Geometry check sheet. Reference: the model listing, model coordinates, mm. Face numbers are marked on the shaded views. A direction names the side the tool comes from. Coordinates: 2 decimals unless noted, no trailing zeros. Order: outer loops, then holes, each group sorted by start corner. A loop starts at its lowest first (then second) coordinate and runs counter-clockwise, first axis right, second up. Notation, with made-up numbers: M 46.25,-38.75 L 88.25,-38.75 A23 cw 88.25,-25.75 Z; hole C 30.5,-19.75 d10. An arc over 180 degrees is marked long. One line per item, written item: value. Start each with the question number.
1) Access from +Z, -Z, +X, -X, +Y, -Y to the whole of each face (thin tool, end or side, straight path). Record for the marked faces 1 and 2.
2) Go/stop test with flat-tipped pins: P1, Ø1, axis at x = -11, z = 11, coming from the -Y side; P2, Ø1, axis at y = 55.5, z = 3, coming from the +X side; P3, Ø7, axis at x = -10.5, z = 8.5, coming from the -Y side; P4, Ø8, axis at x = 5, y = 83, coming from the -Z side. Record where each tip stops, or that it passes through.
3) Draft check along Y on the marked faces 3, 4 and 5. Enter one of: pulls with the +Y half, pulls with the -Y half, needs draft (parallel to the pull), parting line crosses it, or undercut.
4) Sectioned sample at D-D, the plane y = 89. Enter the section's corners in (x, z), then the cut area to 3 significant figures.
5) Sectioned sample at B-B, the plane y = 49. Enter the section's corners in (x, z), then the cut area to 3 significant figures.
6) Sectioned sample at A-A, the plane z = 8.5. Enter the section's corners in (x, y).
7) Thickness scan on L1, parallel to X at y = 16.5, z = 6.25; L2, parallel to X at y = 42.5, z = 4; L3, parallel to X at y = 92.5, z = 11. Record the ranges inside material, lowest first. Write a range as from..to.
8) Sectioned sample at C-C, the plane x = 1. Enter the section's corners in (y, z).
```python
from build123d import *

# Parameters (mm, degrees)
PAD_DEPTH = 13.8


with BuildPart() as part:
    # Sketch → Pad (new body)
    with BuildSketch(Plane.XY):
        with BuildLine():
            Line((-22.5, 100.92), (22.5, 100.92))
            ThreePointArc((49.679403, 64.194795), (45.344368, 89.406544), (22.5, 100.92))
            Line((49.679403, 64.194795), (28.613925, -4.743552))
            ThreePointArc((-28.613925, -4.743552), (0, -25.92), (28.613925, -4.743552))
            Line((-49.679403, 64.194795), (-28.613925, -4.743552))
            ThreePointArc((-22.5, 100.92), (-45.344368, 89.406544), (-49.679403, 64.194795))
        make_face()
        with BuildLine():
            Line((3.825391, 2.831076), (24.890869, 71.769422))
            ThreePointArc((24.890869, 71.769422), (24.972567, 72.130658), (25, 72.5))
            ThreePointArc((25, 72.5), (24.267767, 74.267767), (22.5, 75))
            Line((-22.5, 75), (22.5, 75))
            ThreePointArc((-22.5, 75), (-24.267767, 74.267767), (-25, 72.5))
            ThreePointArc((-25, 72.5), (-24.972567, 72.130658), (-24.890869, 71.769422))
            Line((-3.825391, 2.831076), (-24.890869, 71.769422))
            ThreePointArc((-3.825391, 2.831076), (0, 0), (3.825391, 2.831076))
        make_face(mode=Mode.SUBTRACT)
    extrude(amount=PAD_DEPTH)


solid = part.part
```
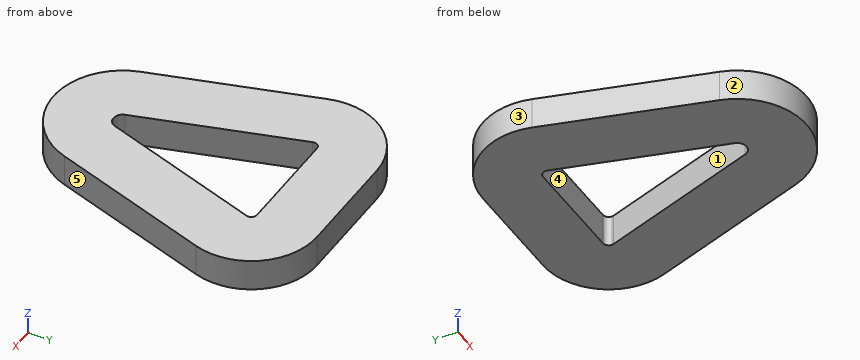
Final values:
1. face 1: +Z, -Z
1. face 2: +Z, -Z, -Y
2. P1: stops at y = -24.02
2. P2: stops at x = 47.18
2. P3: stops at y = -25.09
2. P4: stops at z = 0
3. face 3: parting line crosses it
3. face 4: undercut
3. face 5: pulls with the -Y half
4. outline: M -45.64,0 L 45.64,0 L 45.64,13.8 L -45.64,13.8 Z
4. area: 1,260 mm^2
5. outline: M -45.04,0 L -17.93,0 L -17.93,13.8 L -45.04,13.8 Z; M 17.93,0 L 45.04,0 L 45.04,13.8 L 17.93,13.8 Z
5. area: 748 mm^2
6. outline: M -49.68,64.19 L -28.61,-4.74 A29.92 ccw 28.61,-4.74 L 49.68,64.19 A28.42 ccw 22.5,100.92 L -22.5,100.92 A28.42 ccw Z; hole M -25,72.5 A2.5 ccw -24.89,71.77 L -3.83,2.83 A4 ccw 3.83,2.83 L 24.89,71.77 A2.5 ccw 25,72.5 A2.5 ccw 22.5,75 L -22.5,75 A2.5 ccw Z
7. L1: x = -35.11..-8, 8..35.11
7. L2: x = -43.05..-15.95, 15.95..43.05
7. L3: x = -42.69..42.69
8. outline: M -25.9,0 L 0.13,0 L 0.13,13.8 L -25.9,13.8 Z; M 75,0 L 100.92,0 L 100.92,13.8 L 75,13.8 Z
